```python
from build123d import *

# Parameters (mm, degrees)
BOSS_EXTRUDE1_DEPTH     = 10
BOSS_EXTRUDE2_DEPTH     = 2
SKETCH4_W               = 2
SKETCH4_H               = 2
CUT_EXTRUDE1_DEPTH      = 3.67
FILLET1_R               = 2
CUT_EXTRUDE2_DEPTH      = 13.355398317
CUT_EXTRUDE2_DEPTH_BACK = 13.355398317
SKETCH6_R               = 1.165


with BuildPart() as part:
    # Sketch2 → Boss-Extrude1 (new body)
    with BuildSketch(Plane(origin=(0, 0, 0), x_dir=(1, 0, 0), z_dir=(0, 1, 0))):
        Polygon((-1.835, -2.335), (-1.835, 2.335), (1.835, 2.013916605), (1.835, -2.013916605), align=None)
    extrude(amount=BOSS_EXTRUDE1_DEPTH)

    # Sketch3 → Boss-Extrude2 (add)
    with BuildSketch(Plane(origin=(0, 10, 0), x_dir=(1, 0, 0), z_dir=(0, 1, 0))):
        Polygon((1.835, -2.013916605), (1.835, 2.013916605), (-1.835, 2.335), (-1.835, -2.335), align=None)
    extrude(amount=BOSS_EXTRUDE2_DEPTH)

    # Sketch4 → Cut-Extrude1 (cut)
    with BuildSketch(Plane(origin=(1.835, 0, 0), x_dir=(0, 0, -1), z_dir=(1, 0, 0))):
        with Locations((0, 6)):
            Rectangle(SKETCH4_W, SKETCH4_H)
    extrude(amount=-CUT_EXTRUDE1_DEPTH, mode=Mode.SUBTRACT)

    # Fillet1
    # the kernel refuses this fillet: 2 mm, written as the material it takes off along each edge
    with BuildSketch(Plane(origin=(1.835, 12, 7.013916605), x_dir=(-1, 0, 0), z_dir=(0, 0, -1))) as fillet1_piece_1:
        with BuildLine():
            CenterArc((FILLET1_R, -FILLET1_R), FILLET1_R, 90, 90)
            Line((0, -FILLET1_R), (0, 0))
            Line((0, 0), (FILLET1_R, 0))
        make_face()
    extrude(amount=14.02783321, mode=Mode.SUBTRACT)
    with BuildSketch(Plane(origin=(-1.835, 12, -7.335), x_dir=(0, -1, 0), z_dir=(0, 0, 1))) as fillet1_piece_2:
        with BuildLine():
            CenterArc((FILLET1_R, FILLET1_R), FILLET1_R, 180, 90)
            Line((0, FILLET1_R), (0, 0))
            Line((0, 0), (FILLET1_R, 0))
        make_face()
    extrude(amount=14.67, mode=Mode.SUBTRACT)
    with BuildSketch(Plane(origin=(-1.835, 7, -1), x_dir=(0, 1, 0), z_dir=(0, 0, 1)), Plane(origin=(1.835, 7, -1), x_dir=(-1, 0, 0), z_dir=(0, 0, 1))) as fillet1_piece_3:
        with BuildLine():
            CenterArc((FILLET1_R, -FILLET1_R), FILLET1_R, 90, 90)
            Line((0, -FILLET1_R), (0, 0))
            Line((0, 0), (FILLET1_R, 0))
        make_face()
    extrude(amount=2, mode=Mode.SUBTRACT)

    # Sketch6 → Cut-Extrude2 (cut, two sides: drawn at the far end of the back side and taken through both)
    with BuildSketch(Plane.XY.offset(-CUT_EXTRUDE2_DEPTH_BACK)):
        with Locations((0, 3)):
            Circle(SKETCH6_R)
    extrude(amount=CUT_EXTRUDE2_DEPTH + CUT_EXTRUDE2_DEPTH_BACK, mode=Mode.SUBTRACT)


solid = part.part
```
Geometry: final body of the model. Coordinates: model frame, mm. A direction names the side the tool comes from. Coordinates: 2 decimals unless noted, no trailing zeros. Order: outer loops, then holes, each group sorted by start corner. A loop starts at its lowest first (then second) coordinate and runs counter-clockwise, first axis right, second up. Notation, with made-up numbers: (53.5, 75.5) -> (103.5, 75.5) arc R15 cw to (103.5, 99.5) -> close; hole circle Ø11 at (-22, 38.5). An arc over 180 degrees is marked (long way). Write each question's results on one line, items separated by ' | '. Start each with the question number.
1) Cut plane B-B, the plane y = 5.75. Output: boundary loops of the cut face in (x, z) (3 decimals).
2) Mould query, pull axis Z, two halves, no side actions, for faces 1 (the flat face through (-0.026, 5.913, 2.177)), 2 (the flat face through (0, 6, 1)), 3 (the cylindrical face through (1.29, 11.37, 0.03)), 4 (the flat face through (0.03, 5.91, -2.17)). Classes: released by +Z, released by -Z, zero draft, split by the parting line, or undercut.
3) Cut plane D-D, the plane z = 1.5. Output: boundary loops of the cut face in (x, y) (3 decimals).
4) Cut plane C-C, the plane x = 0.8. Output: boundary loops of the cut face in (y, z).
5) Set-up query: faces 5 (the flat face through (0, 5, 0)), 6 (the cylindrical face through (1.29, 7.63, -0.01)), 7 (the cylindrical face through (-1.32, 7.66, -0.01)), 8 (the flat face through (0, 0, 0)). Return all of +Z, -Z, +X, -X, +Y, -Y with unobstructed straight access to the full face (end or side cutting, diameter ignored); none if empty.
6) First-contact query: pin 1 (1.5 mm diameter, centred on x = -0.5, y = 1.5, fed in from -Z); pin 2 (2 mm diameter, centred on x = 0, y = 3, fed in from +Z); pin 3 (1.8 mm diameter, centred on x = 0.5, y = 6.5, fed in from +Z); pin 4 (1 mm diameter, centred on x = 1, y = 8.5, fed in from +Z). Flat tips, straight axial feed; report the tip coordinate or a pass-through.
7) Cut plane A-A, the plane z = 0.4. Output: boundary loops of the cut face in (x, y) (3 decimals).
8) Material intervals for line 1 along X through (y, z) = (3, -1.25) (3 decimals); line 2 along Y through (x, z) = (-0.95, 0.6); line 3 along Y through (x, z) = (0.2, 1.55), sorted ascending.
Checks:
1) outline: (-1.835, -2.335) -> (1.835, -2.014) -> (1.835, -1) -> (-1.835, -1) -> close; (-1.835, 1) -> (1.835, 1) -> (1.835, 2.014) -> (-1.835, 2.335) -> close
2) face 1: released by +Z | face 2: undercut | face 3: zero draft | face 4: released by -Z
3) outline: (-1.835, 0) -> (1.835, 0) -> (1.835, 10) arc R2 ccw to (0, 11.993) arc R2 ccw to (-1.835, 10) -> close; hole circle Ø2.33 at (0, 3)
4) outline: (0, -2.1) -> (2.15, -2.1) -> (2.15, 2.1) -> (0, 2.1) -> close; (3.85, -2.1) -> (11.75, -2.1) -> (11.75, 2.1) -> (3.85, 2.1) -> close; hole (5, -1) -> (7.25, -1) -> (7.25, 1) -> (5, 1) -> close
5) face 5: +X, -X | face 6: +X | face 7: -X | face 8: +Z, -Z, +X, -X, -Y
6) pin 1: z = -2.28 | pin 2: through | pin 3: z = 2.21 | pin 4: z = 2.13
7) outline: (-1.835, 0) -> (1.835, 0) -> (1.835, 5) -> (-1.835, 5) -> close; (-1.835, 9) arc R2 ccw to (0, 7.007) arc R2 ccw to (1.835, 9) -> (1.835, 10) arc R2 ccw to (0, 11.993) arc R2 ccw to (-1.835, 10) -> close; hole circle Ø2.33 at (0, 3)
8) line 1: -1.835 to -1.165, 1.165 to 1.835 | line 2: 0 to 2.33, 3.67 to 5, 7.34 to 11.66 | line 3: 0 to 1.85, 4.15 to 11.97
